Source: CAD feature listing. Evaluate the final solid. Frame: model axes, mm. A direction names the side the tool comes from. Round coordinates to 2 decimals unless told otherwise and drop trailing zeros. Loops run counter-clockwise (first coordinate to the right, second up) from the corner with the lowest first, then second, coordinate; pieces in that order, holes last. Notation, with made-up numbers: M 86,67.5 L 144,67.5 A22 ccw 144,99.5 Z; hole C 56,4.25 d10. An arc over 180 degrees is marked long. Answer as CSV lines item,"result". Start each with the question number.
```python
from build123d import *

# Parameters (mm, degrees)
SKETCH1_R           = 25
BOSS_EXTRUDE1_DEPTH = 30
SKETCH2_R           = 10
BOSS_EXTRUDE2_DEPTH = 20
SKETCH3_R           = 7.5
CUT_EXTRUDE1_DEPTH  = 20
SKETCH4_R           = 5
BOSS_EXTRUDE3_DEPTH = 30
SKETCH5_R           = 7.5
BOSS_EXTRUDE4_DEPTH = 5
SKETCH7_W           = 10
SKETCH7_H           = 5
BOSS_EXTRUDE5_DEPTH = 10
SKETCH8_R           = 3.75
CUT_EXTRUDE2_DEPTH  = 5
CUT_EXTRUDE3_START  = -5
SKETCH9_R           = 3.75
CUT_EXTRUDE3_DEPTH  = 5
FILLET1_R           = 5
FILLET2_R           = 5
FILLET3_R           = 1


# Some blends are built 0.0001 mm under size
with BuildPart() as part:
    # Sketch1 → Boss-Extrude1 (new body)
    with BuildSketch(Plane.XY):
        Circle(SKETCH1_R)
    extrude(amount=BOSS_EXTRUDE1_DEPTH)

    # Sketch2 → Boss-Extrude2 (add)
    with BuildSketch(Plane.XY.offset(30)):
        Circle(SKETCH2_R)
    extrude(amount=BOSS_EXTRUDE2_DEPTH)

    # Sketch3 → Cut-Extrude1 (cut)
    with BuildSketch(Plane.XY.offset(50)):
        Circle(SKETCH3_R)
    extrude(amount=-CUT_EXTRUDE1_DEPTH, mode=Mode.SUBTRACT)

    # Sketch4 → Boss-Extrude3 (add)
    with BuildSketch(Plane.XY.offset(30)):
        Circle(SKETCH4_R)
    extrude(amount=BOSS_EXTRUDE3_DEPTH)

    # Sketch5 → Boss-Extrude4 (add)
    with BuildSketch(Plane(origin=(0, 0, 0), x_dir=(-1, 0, 0), z_dir=(0, 0, -1))):
        with Locations(Location((0, 0, 0), (0, 0, 180))):
            Circle(SKETCH5_R)
    extrude(amount=BOSS_EXTRUDE4_DEPTH)

    # Sketch7 → Boss-Extrude5 (add)
    with BuildSketch(Plane(origin=(0, 0, 0), x_dir=(-1, 0, 0), z_dir=(0, 0, -1))):
        with Locations((0, 17.5)):
            Rectangle(SKETCH7_W, SKETCH7_H)
        with Locations((0, -17.5)):
            Rectangle(SKETCH7_W, SKETCH7_H)
    extrude(amount=BOSS_EXTRUDE5_DEPTH)

    # Sketch8 → Cut-Extrude2 (cut)
    with BuildSketch(Plane(origin=(0, 20, 0), x_dir=(1, 0, 0), z_dir=(0, 1, 0))):
        with Locations(Location((0, 5, 0), (0, 0, 180))):
            Circle(SKETCH8_R)
    extrude(amount=-CUT_EXTRUDE2_DEPTH, mode=Mode.SUBTRACT)

    # Sketch9 → Cut-Extrude3 (cut)
    with BuildSketch(Plane(origin=(0, -20, 0), x_dir=(-1, 0, 0), z_dir=(0, -1, 0)).offset(CUT_EXTRUDE3_START)):
        with Locations((0, 5)):
            Circle(SKETCH9_R)
    extrude(amount=CUT_EXTRUDE3_DEPTH, mode=Mode.SUBTRACT)

    # Fillet1
    # the kernel refuses this fillet: 5 mm, written as the material it takes off along each edge
    with BuildSketch(Plane(origin=(0, 0, 30), x_dir=(1, 0, 0), z_dir=(0, -1, 0))) as fillet1_piece_1:
        with BuildLine():
            CenterArc((25 - FILLET1_R, -FILLET1_R), FILLET1_R, 0, 90)
            Line((25 - FILLET1_R, 0), (25, 0))
            Line((25, 0), (25, -FILLET1_R))
        make_face()
    revolve(axis=Axis((0, 0, 30), (0, 0, 1)), mode=Mode.SUBTRACT)
    with BuildSketch(Plane(origin=(0, 0, 0), x_dir=(1, 0, 0), z_dir=(0, -1, 0))) as fillet1_piece_2_section:
        with BuildLine():
            CenterArc((25 - FILLET1_R, FILLET1_R), FILLET1_R, 270, 90)
            Line((25 - FILLET1_R, 0), (25, 0))
            Line((25, 0), (25, FILLET1_R))
        make_face()
    fillet1_piece_2 = revolve(axis=Axis((0, 0, 0), (0, 0, 1)), mode=Mode.PRIVATE)
    fillet1_piece_2 = split(fillet1_piece_2, bisect_by=Plane(origin=(5, 14.511659558, 1.419610571), z_dir=(1, 0, 0)), keep=Keep.TOP, mode=Mode.PRIVATE)
    add(fillet1_piece_2, mode=Mode.SUBTRACT)
    with BuildSketch(Plane(origin=(0, 0, 0), x_dir=(1, 0, 0), z_dir=(0, -1, 0))) as fillet1_piece_3_section:
        with BuildLine():
            CenterArc((25 - FILLET1_R, FILLET1_R), FILLET1_R, 270, 90)
            Line((25 - FILLET1_R, 0), (25, 0))
            Line((25, 0), (25, FILLET1_R))
        make_face()
    fillet1_piece_3 = revolve(axis=Axis((0, 0, 0), (0, 0, 1)), mode=Mode.PRIVATE)
    fillet1_piece_3 = split(fillet1_piece_3, bisect_by=Plane(origin=(4.6e-08, 20, 1.116734198), z_dir=(0, 1, 0)), keep=Keep.TOP, mode=Mode.PRIVATE)
    add(fillet1_piece_3, mode=Mode.SUBTRACT)
    with BuildSketch(Plane(origin=(0, 0, 0), x_dir=(1, 0, 0), z_dir=(0, -1, 0))) as fillet1_piece_4_section:
        with BuildLine():
            CenterArc((25 - FILLET1_R, FILLET1_R), FILLET1_R, 270, 90)
            Line((25 - FILLET1_R, 0), (25, 0))
            Line((25, 0), (25, FILLET1_R))
        make_face()
    fillet1_piece_4 = revolve(axis=Axis((0, 0, 0), (0, 0, 1)), mode=Mode.PRIVATE)
    fillet1_piece_4 = split(fillet1_piece_4, bisect_by=Plane(origin=(-4.6e-08, -20, 1.116734198), z_dir=(0, -1, 0)), keep=Keep.TOP, mode=Mode.PRIVATE)
    add(fillet1_piece_4, mode=Mode.SUBTRACT)
    with BuildSketch(Plane(origin=(0, 0, 0), x_dir=(1, 0, 0), z_dir=(0, -1, 0))) as fillet1_piece_5_section:
        with BuildLine():
            CenterArc((25 - FILLET1_R, FILLET1_R), FILLET1_R, 270, 90)
            Line((25 - FILLET1_R, 0), (25, 0))
            Line((25, 0), (25, FILLET1_R))
        make_face()
    fillet1_piece_5 = revolve(axis=Axis((0, 0, 0), (0, 0, 1)), mode=Mode.PRIVATE)
    fillet1_piece_5 = split(fillet1_piece_5, bisect_by=Plane(origin=(-5, 0, 1.419610538), z_dir=(-1, 0, 0)), keep=Keep.TOP, mode=Mode.PRIVATE)
    add(fillet1_piece_5, mode=Mode.SUBTRACT)

    # Fillet2
    fillet2_edges = [part.edges().sort_by_distance(p)[0] for p in [
        (5, -17.5, -10),
        (-5, -17.5, -10),
        (5, 17.5, -10),
        (-5, 17.5, -10),
    ]]
    fillet(fillet2_edges, radius=FILLET2_R - 0.0001)  # a hair under: the kernel refuses the full size

    # Fillet3
    fillet3_edges = [part.edges().sort_by_distance(p)[0] for p in [
        (-7.5, 0, 0),
        (-7.5, 0, -5),
    ]]
    fillet(fillet3_edges, radius=FILLET3_R)


solid = part.part
```
1) Access query for faces 5 (the cylindrical face through (-7.493, 0.33, 40.14)), 6 (the flat face through (9, 0, 0)), 7 (the cylindrical face through (0.81, -17.46, -1.34)), 8 (the flat face through (0, 0, -5)), 9 (the flat face through (5, -18, -3)). Directions: +Z, -Z, +X, -X, +Y, -Y. A direction counts if a zero-diameter tool reaches every point of the face in a straight line with its end or side. Return the directions, or none.
2) Section B-B, the plane z = 45.5. Return loops of the section in (x, y).
3) Section A-A, the plane y = 0. Return loops of the section in (x, z), and give its area (3 significant figures).
4) Section D-D, the plane z = 17. Return loops of the section in (x, y), and give its area (3 significant figures).
5) Ray query, line 1 along Y through (x, z) = (0, 42.25); line 2 along Z through (x, y) = (0, 18.9); line 3 along X through (y, z) = (-18.3, -5). Return the intervals inside material, ascending.
6) Section C-C, the plane z = 53. Return loops of the section in (x, y).
7) Contact query for flat-ended pins moving along their axis: pin 1 Ø2.5 at (y, z) = (-16.5, -3.5) entering from +X; pin 2 Ø10 at (y, z) = (2, 47.5) entering from +X; pin 3 Ø4 at (x, y) = (1.5, -3) entering from -Z; pin 4 Ø1.5 at (x, y) = (4.5, 2.5) entering from +Z. Output: stop coordinate, or through.
8) Mould query, pull axis Z, two halves, no side actions, for faces 1 (the cylindrical face through (0.81, 17.54, -8.66)), 2 (the flat face through (4, 7, 50)), 3 (the cylindrical face through (-3, -17, -9)), 4 (the cylindrical face through (4.032, -6.324, -2.479)). Classes: pulls with the +Z half, pulls with the -Z half, needs draft (parallel to the pull), parting line crosses it, or undercut.
Findings below:
1,face 5,"+Z"
1,face 6,"-Z"
1,face 7,"-Y"
1,face 8,"-Z, +X, -X"
1,face 9,"-Z, +X, -Y"
2,outline,"C 0,0 d20; C 0,0 d10; hole C 0,0 d15"
3,outline,"M -25,5 A5 ccw -20,0 L -8.5,0 A1 cw -7.5,-1 L -7.5,-4 A1 ccw -6.5,-5 L 6.5,-5 A1 ccw 7.5,-4 L 7.5,-1 A1 cw 8.5,0 L 20,0 A5 ccw 25,5 L 25,25 A5 ccw 20,30 L 10,30 L 10,50 L 7.5,50 L 7.5,30 L 5,30 L 5,60 L -5,60 L -5,30 L -7.5,30 L -7.5,50 L -10,50 L -10,30 L -20,30 A5 ccw -25,25 Z"
3,area,"1,950 mm²"
4,outline,"C 0,0 d50"
4,area,"1,960 mm²"
5,line 1,"-10 to -7.5, -5 to 5, 7.5 to 10"
5,line 2,"-10 to -8.75, -1.25 to 30"
5,line 3,"-5 to -3.75, 3.75 to 5"
6,outline,"C 0,0 d10"
7,pin 1,"x = 5"
7,pin 2,"x = 10"
7,pin 3,"z = -5"
7,pin 4,"z = 60"
8,face 1,"undercut"
8,face 2,"pulls with the +Z half"
8,face 3,"pulls with the -Z half"
8,face 4,"needs draft"
